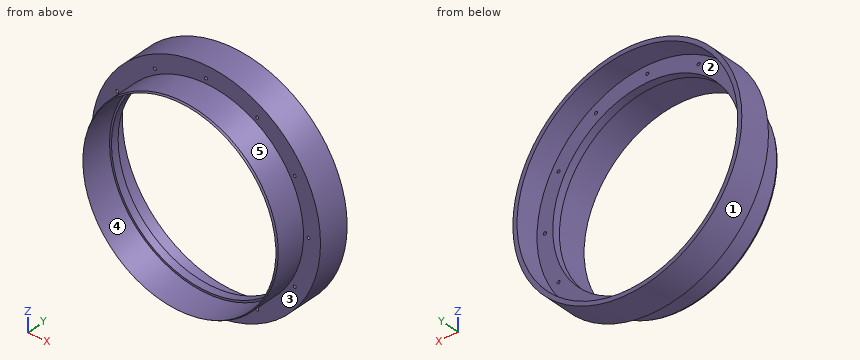
```python
from build123d import *

# Parameters (mm, degrees)
SCREW_HOLES_COUNT = 12


with BuildPart() as part:
    # Cross Section → Main (revolve)
    with BuildSketch(Plane.XY):
        Polygon((-38.1, 0), (-38.1, -3.175), (-38.8874, -3.175), (-38.8874, -15.875), (-39.2684, -15.215088642), (-39.2684, -3.175), (-46.1264, -3.175), (-46.1264, 9.525), (-44.45, 9.525), (-44.45, 0), align=None)
    revolve(axis=Axis((0, 55, 0), (0, -1, 0)))

    # Sketch7 → #0-80 Tapped Hole1 (revolve, cut)
    with BuildSketch(Plane(origin=(-41.275, 0, 0), x_dir=(0, 0, 1), z_dir=(1, 0, 0))):
        Polygon((0, 0), (0, 3.532890611), (0.59563, 3.175), (0.59563, 0), align=None)
    f_0_80_tapped_hole1 = revolve(axis=Axis((-41.275, 6.35, 0), (0, -1, 0)), mode=Mode.SUBTRACT)

    # Screw Holes: #0-80 Tapped Hole1 ×12 about axis
    screw_holes_axis = Axis((0, 0, 0), (0, 1, 0))
    for i in range(1, SCREW_HOLES_COUNT):
        add(f_0_80_tapped_hole1.rotate(screw_holes_axis, i * 360 / SCREW_HOLES_COUNT), mode=Mode.SUBTRACT)


solid = part.part
```
The listing builds one solid part. Answer for the finished solid, in the listing's coordinates (mm). Face numbers are marked on the shaded views. A direction names the side the tool comes from. Coordinates: 2 decimals unless noted, no trailing zeros. Write each loop counter-clockwise with the first axis right and the second up, starting at its lowest first coordinate (ties: lowest second). Pieces come first, ordered by that corner, then holes.
Q1. The mould has two halves that part along Z. Classify the marked faces 3, 4 and 5: released by +Z, released by -Z, zero draft, split by the parting line, or undercut.
Returned:
face 3: zero draft
face 4: undercut
face 5: split by the parting line
Q2. Given P1, Ø4, axis at x = 0.5, y = -8, coming from the +Z side; P2, Ø1.9, axis at x = 0, z = 41.275, coming from the -Y side (3 decimals); P3, Ø2, axis at x = -35.5, y = -5, coming from the -Z side, each flat-ended and moving along its own axis, determine where each tip first touches the part or whether it passes through.
Returned:
P1: stops at z = 39.27
P2: stops at y = -3.175
P3: stops at z = -18.76
Q3. Section B-B, the plane y = -10.5 is taken. Write down the section's boundary in (x, z), then the cut area to 3 significant figures.
Returned:
outline: circle Ø78.54 at (0, 0); hole circle Ø77.77 at (0, 0)
area: 93.5 mm2
Q4. Find the intervals of material crossed by line 1 along Z through (x, y) = (0.5, 6.5); line 2 along X through (y, z) = (-13, 0); line 3 along X through (y, z) = (-0.65, 0), in increasing order.
Returned:
line 1: z = -46.12 to -44.45, 44.45 to 46.12
line 2: x = -39.27 to -38.89, 38.89 to 39.27
line 3: x = -46.13 to -41.87, -40.68 to -38.1, 38.1 to 40.68, 41.87 to 46.13
Q5. Which of the six approach directions +Z, -Z, +X, -X, +Y, -Y give full straight-line access (tool end or side, diameter ignored) to the marked faces 1 and 2?
Returned:
face 1: +Y, -Y
face 2: +Y
Q6. Section A-A, the plane y = 5.25 is taken. Write down the section's boundary in (x, z).
Returned:
outline: circle Ø92.25 at (0, 0); hole circle Ø88.9 at (0, 0)
